Input: part model. Units: mm. Frame: model coordinates. A direction names the side the tool comes from. Round coordinates to 2 decimals unless told otherwise and drop trailing zeros. Order: outer loops, then holes, each group sorted by start corner. A loop starts at its lowest first (then second) coordinate and runs counter-clockwise, first axis right, second up. Notation, with made-up numbers: (86, -18.5) -> (139, -18.5) arc R28 cw to (139, 13.5) -> close; hole circle Ø2 at (44, 85.25). An arc over 180 degrees is marked (long way). Use a Markdown table: item, result.
from build123d import *

# Parameters (mm, degrees)
PAD_DEPTH            = 6.5
POCKET_DEPTH         = 6
SKETCH002_R          = 13.5
POCKET001_DEPTH      = 1
SKETCH003_W          = 5.45
SKETCH003_H          = 6.5
PAD001_DEPTH         = 3.5
POCKET002_DEPTH      = 10
SKETCH010_W          = 4
SKETCH010_H          = 6.5
PAD002_DEPTH         = 3.5
POCKET005_DEPTH      = 10
SKETCH015_R          = 2.2
SKETCH015_R_2        = 1.025
PAD003_DEPTH         = 2
POCKET009_DEPTH      = 4
POCKET010_DEPTH      = 4
PAD004_DEPTH         = 4
POCKET013_DEPTH      = 12.201
POCKET013_DEPTH_BACK = 36.201
SKETCH022_R          = 0.6
POCKET014_DEPTH      = 2
SKETCH023_R          = 0.6
POCKET015_DEPTH      = 2
SKETCH024_R          = 13.5
PAD005_DEPTH         = 1
SKETCH025_R          = 20.45
SKETCH025_R_2        = 19.85
POCKET016_DEPTH      = 0.3
SKETCH026_R          = 1
POCKET017_DEPTH      = 5
SKETCH027_W          = 5.4500000001
SKETCH027_H          = 2
SKETCH027_W_2        = 5.45
PAD006_DEPTH         = 2


with BuildPart() as part:
    # Sketch → Pad (new body)
    with BuildSketch(Plane.XY):
        with BuildLine():
            Line((-22.5019915649, 16), (-22.5019915649, -16))
            Line((-22.5019915649, -16), (-16.2858834578, -17.9))
            ThreePointArc((-16.2858834578, -17.9), (-0.4552796053, -24.1957169863), (15.6009615088, -18.5))
            Line((15.6009615088, -18.5), (24.5395016581, -17.45))
            Line((24.5395016581, 17.45), (24.5395016581, -17.45))
            Line((15.6009615088, 18.5), (24.5395016581, 17.45))
            ThreePointArc((15.6009615088, 18.5), (-0.4552796053, 24.1957169863), (-16.2858834578, 17.9))
            Line((-22.5019915649, 16), (-16.2858834578, 17.9))
        make_face()
    extrude(amount=PAD_DEPTH)

    # Sketch001 → Pocket (cut)
    with BuildSketch(Plane.XY):
        with BuildLine():
            Line((-14.8539557021, 16.9), (-21.2122180433, 15.55))
            Line((-21.2122180433, 15.55), (-21.2122180433, -15.55))
            Line((-21.2122180433, -15.55), (-14.8539557021, -16.9))
            ThreePointArc((-14.8539557021, -16.9), (-0.0760301383, -22.4998715423), (14.739402973, -17))
            Line((14.739402973, -17), (23.6191552218, -16.4))
            Line((23.6191552218, 16.4), (23.6191552218, -16.4))
            Line((14.739402973, 17), (23.6191552218, 16.4))
            ThreePointArc((14.739402973, 17), (-0.0760301383, 22.4998715423), (-14.8539557021, 16.9))
        make_face()
    extrude(amount=POCKET_DEPTH, mode=Mode.SUBTRACT)

    # Sketch002 (on Face19 of Pocket) → Pocket001 (cut)
    with BuildSketch(Plane(origin=(0, 0, 6), x_dir=(1, 0, 0), z_dir=(0, 0, -1))):
        Circle(SKETCH002_R)
    extrude(amount=-POCKET001_DEPTH, mode=Mode.SUBTRACT)

    # Sketch003 (on Face7 of Pad) → Pad001 (join)
    with BuildSketch(Plane.YZ.offset(24.5395016581)):
        with Locations((-14.725, 3.25)):
            Rectangle(SKETCH003_W, SKETCH003_H)
        with Locations((14.725, 3.25)):
            Rectangle(SKETCH003_W, SKETCH003_H)
    extrude(amount=PAD001_DEPTH)

    # Sketch006 (on Face22 of Pad001) → Pocket002 (cut)
    with BuildSketch(Plane.XY.offset(6.5)):
        with BuildLine():
            ThreePointArc((24.5395016581, 17.45), (26.1592830786, 16.2095505764), (28.0395016581, 15.4176006311))
            Line((28.0395016581, 17.45), (28.0395016581, 15.4176006311))
            Line((28.0395016581, 17.45), (24.5395016581, 17.45))
        make_face()
        with BuildLine():
            ThreePointArc((28.0395016581, -15.4176006311), (26.1592830786, -16.2095505765), (24.5395016581, -17.4500000001))
            Line((28.0395016581, -17.45), (24.5395016581, -17.4500000001))
            Line((28.0395016581, -15.4176006311), (28.0395016581, -17.45))
        make_face()
    extrude(amount=-POCKET002_DEPTH, mode=Mode.SUBTRACT)

    # Sketch010 (on Face3 of Pad) → Pad002 (join)
    with BuildSketch(Plane(origin=(-22.5019915649, 0, 0), x_dir=(0, -1, 0), z_dir=(-1, 0, 0))):
        with Locations((-14, 3.25)):
            Rectangle(SKETCH010_W, SKETCH010_H)
        with Locations((14, 3.25)):
            Rectangle(SKETCH010_W, SKETCH010_H)
    extrude(amount=PAD002_DEPTH)

    # Sketch011 (on Face28 of Pad002) → Pocket005 (cut)
    with BuildSketch(Plane.XY.offset(6.5)):
        Polygon((-26.0019915649, 16), (-22.5019915649, 16), (-26.0019915649, 14.5), align=None)
        Polygon((-22.5019915649, -16), (-26.0019915649, -14.5), (-26.0019915649, -16), align=None)
    extrude(amount=-POCKET005_DEPTH, mode=Mode.SUBTRACT)

    # Sketch015 (on Face19 of Pocket) → Pad003 (join)
    with BuildSketch(Plane(origin=(0, 0, 6), x_dir=(1, 0, 0), z_dir=(0, 0, -1))):
        with Locations((-18.42, 13.32)):
            Circle(SKETCH015_R)
        with Locations((-18.42, 13.32)):
            Circle(SKETCH015_R_2, mode=Mode.SUBTRACT)
        with Locations((7.27, 18.56)):
            Circle(SKETCH015_R)
        with Locations((7.27, 18.56)):
            Circle(SKETCH015_R_2, mode=Mode.SUBTRACT)
        with Locations((5.37, -19.79)):
            Circle(SKETCH015_R)
        with Locations((5.37, -19.79)):
            Circle(SKETCH015_R_2, mode=Mode.SUBTRACT)
        with Locations((-18.42, -13.32)):
            Circle(SKETCH015_R)
        with Locations((-18.42, -13.32)):
            Circle(SKETCH015_R_2, mode=Mode.SUBTRACT)
    extrude(amount=PAD003_DEPTH)

    # Sketch016 (on Face4 of Pocket) → Pocket009 (cut)
    with BuildSketch(Plane(origin=(0, 0, 0), x_dir=(1, 0, 0), z_dir=(0, 0, -1))):
        with BuildLine():
            Line((-4.9992330338, 23.6779996848), (-5.0007669662, 21.9372361465))
            ThreePointArc((5.0007669662, 21.9372361465), (0, 22.5), (-5.0007669662, 21.9372361465))
            Line((5.0007669662, 23.6776757675), (5.0007669662, 21.9372361465))
            ThreePointArc((5.0007669662, 23.6776757675), (0.00078388, 24.1999999873), (-4.9992330338, 23.6779996848))
        make_face()
    extrude(amount=-POCKET009_DEPTH, mode=Mode.SUBTRACT)

    # Sketch017 (on Face4 of Pocket) → Pocket010 (cut)
    with BuildSketch(Plane(origin=(0, 0, 0), x_dir=(1, 0, 0), z_dir=(0, 0, -1))):
        with BuildLine():
            ThreePointArc((-3.2541322314, -22.2634369184), (0, -22.5), (3.2541322314, -22.2634369184))
            Line((3.2541322314, -22.2634369184), (3.5, -23.9455632634))
            ThreePointArc((-3.5, -23.9455632634), (0, -24.2), (3.5, -23.9455632634))
            Line((-3.2541322314, -22.2634369184), (-3.5, -23.9455632634))
        make_face()
        with BuildLine():
            ThreePointArc((-13.9498796389, -17.6536358312), (-11.25, -19.4855715851), (-8.3135572795, -20.9077680626))
            Line((-8.3135572795, -20.9077680626), (-8.9416927184, -22.487466094))
            ThreePointArc((-15.0038705449, -18.987466094), (-12.1, -20.9578147716), (-8.9416927184, -22.487466094))
            Line((-13.9498796389, -17.6536358312), (-15.0038705449, -18.987466094))
        make_face()
        with BuildLine():
            ThreePointArc((8.3135572795, -20.9077680626), (11.25, -19.4855715851), (13.9498796389, -17.6536358312))
            Line((13.9498796389, -17.6536358312), (15.0038705449, -18.987466094))
            ThreePointArc((8.9416927184, -22.487466094), (12.1, -20.9578147716), (15.0038705449, -18.987466094))
            Line((8.3135572795, -20.9077680626), (8.9416927184, -22.487466094))
        make_face()
    extrude(amount=-POCKET010_DEPTH, mode=Mode.SUBTRACT)

    # Sketch018 (on Face8 of Pocket005) → Pad004 (join)
    with BuildSketch(Plane(origin=(0, 0, 0), x_dir=(1, 0, 0), z_dir=(0, 0, -1))):
        Polygon((-26.0019915649, 14.5), (-26.0019915649, 12), (-22.5019915649, 12), (-22.5019915649, 16), align=None)
        Polygon((-26.0019915649, -12), (-22.5019915649, -12), (-22.5019915649, -16), (-26.0019915649, -14.5), align=None)
        with BuildLine():
            Line((24.5395016581, 17.4500000001), (24.5395016581, 12))
            Line((28.0395016581, 12), (24.5395016581, 12))
            Line((28.0395016581, 15.4176006311), (28.0395016581, 12))
            ThreePointArc((24.5395016581, 17.4500000001), (26.1592830786, 16.2095505765), (28.0395016581, 15.4176006311))
        make_face()
        with BuildLine():
            Line((24.5395016581, -12), (24.5395016581, -17.45))
            ThreePointArc((28.0395016581, -15.4176006311), (26.1592830786, -16.2095505764), (24.5395016581, -17.45))
            Line((28.0395016581, -12), (28.0395016581, -15.4176006311))
            Line((24.5395016581, -12), (28.0395016581, -12))
        make_face()
    extrude(amount=PAD004_DEPTH)

    # Sketch021 (on Face50 of Pad004) → Pocket013 (cut, two sides)
    with BuildSketch(Plane(origin=(0, -12, 0), x_dir=(-1, 0, 0), z_dir=(0, 1, 0))) as pocket013_sk:
        with BuildLine():
            Line((-24.5395016581, -4), (-24.5395016581, -3))
            ThreePointArc((-25.5395016581, -4), (-24.958362828, -3.5811388301), (-24.5395016581, -3))
            Line((-24.5395016581, -4), (-25.5395016581, -4))
        make_face()
        with BuildLine():
            Line((22.5019915649, -4), (22.5019915649, -3))
            ThreePointArc((22.5019915649, -3), (22.9208527349, -3.5811388301), (23.5019915649, -4))
            Line((22.5019915649, -4), (23.5019915649, -4))
        make_face()
        with BuildLine():
            Line((-28.0395016581, 0), (-28.0395016581, 6.5))
            Line((-28.0395016581, 6.5), (-24.5395016581, 6.5))
            ThreePointArc((-24.5395016581, 6.5), (-27.1088837932, 3.6912057651), (-28.0395016581, 0))
        make_face()
        with BuildLine():
            Line((26.0019915649, 6.5), (26.0019915649, 0))
            ThreePointArc((26.0019915649, 0), (25.0713737, 3.6912057651), (22.5019915649, 6.5))
            Line((26.0019915649, 6.5), (22.5019915649, 6.5))
        make_face()
    extrude(amount=-POCKET013_DEPTH, mode=Mode.SUBTRACT)
    extrude(pocket013_sk.sketch, amount=POCKET013_DEPTH_BACK, mode=Mode.SUBTRACT)

    # Sketch022 (on Face66 of Pocket013) → Pocket014 (cut)
    with BuildSketch(Plane.XZ.offset(-12)):
        with Locations((-24.7019915649, -2.7)):
            Circle(SKETCH022_R)
        with Locations((26.7395016581, -2.7)):
            Circle(SKETCH022_R)
    extrude(amount=-POCKET014_DEPTH, mode=Mode.SUBTRACT)

    # Sketch023 (on Face49 of Pocket014) → Pocket015 (cut)
    with BuildSketch(Plane(origin=(0, -12, 0), x_dir=(-1, 0, 0), z_dir=(0, 1, 0))):
        with Locations((-26.7395016581, -2.7)):
            Circle(SKETCH023_R)
        with Locations((24.7019915649, -2.7)):
            Circle(SKETCH023_R)
    extrude(amount=-POCKET015_DEPTH, mode=Mode.SUBTRACT)

    # Sketch024 (on Face16 of Pocket015) → Pad005 (join)
    with BuildSketch(Plane.XY.offset(6.5)):
        with BuildLine():
            ThreePointArc((-22.5019915649, -8.9050758341), (24.2, 0), (-22.5019915649, 8.9050758341))
            Line((-22.5019915649, 8.9050758341), (-22.5019915649, -8.9050758341))
        make_face()
        Circle(SKETCH024_R, mode=Mode.SUBTRACT)
    extrude(amount=PAD005_DEPTH)

    # Sketch025 (on Face42 of Pad005) → Pocket016 (cut)
    with BuildSketch(Plane.XY.offset(7.5)):
        Circle(SKETCH025_R)
        Circle(SKETCH025_R_2, mode=Mode.SUBTRACT)
    extrude(amount=-POCKET016_DEPTH, mode=Mode.SUBTRACT)

    # Sketch026 (on DatumPlane) → Pocket017 (cut)
    with BuildSketch(Plane.XZ.offset(25)):
        with Locations((-6.5, 4.8)):
            Circle(SKETCH026_R)
    extrude(amount=-POCKET017_DEPTH, mode=Mode.SUBTRACT)

    # Sketch027 (on Face18 of Pocket017) → Pad006 (join)
    with BuildSketch(Plane(origin=(24.5395016581, 0, 0), x_dir=(0, -1, 0), z_dir=(-1, 0, 0))):
        with Locations((14.7250000001, -2)):
            Rectangle(SKETCH027_W, SKETCH027_H)
        with Locations((-14.725, -2)):
            Rectangle(SKETCH027_W_2, SKETCH027_H)
    extrude(amount=PAD006_DEPTH)


solid = part.part
1) Set-up query: faces 1 (the face through (-8.623, 21.687, 1.972)), 2 (the face through (4.61, 19.1, 5.01)), 3 (the face through (-17, 11, 7.2)), 4 (the face through (22.54, 15, -2)), 5 (the face through (-14.47, 18.31, 1.97)). Return all of +Z, -Z, +X, -X, +Y, -Y with unobstructed straight access to the full face (end or side cutting, diameter ignored); none if empty.
Answer key:
| item | result |
|---|---|
| face 1 | -Z, -X |
| face 2 | -Z |
| face 3 | +Z |
| face 4 | -Z, +Y, -Y |
| face 5 | -Z, +Y |
2) Cut plane B-B on y = -3. Return loops of the section in (x, z), and give its area (3 significant figures).
Answer key:
| item | result |
|---|---|
| outline | (-22.5, 0) -> (-21.21, 0) -> (-21.21, 6) -> (-13.16, 6) -> (-13.16, 7.5) -> (-19.62, 7.5) -> (-19.62, 7.2) -> (-20.23, 7.2) -> (-20.23, 7.5) -> (-22.5, 7.5) -> close; (13.16, 6) -> (23.62, 6) -> (23.62, 0) -> (24.54, 0) -> (24.54, 6.5) -> (24.01, 6.5) -> (24.01, 7.5) -> (20.23, 7.5) -> (20.23, 7.2) -> (19.62, 7.2) -> (19.62, 7.5) -> (13.16, 7.5) -> close |
| area | 43.4 mm^2 |
3) Ray query, probe 1 along Y at (x, z) = (7.27, 5) (3 decimals); probe 2 along Y at (x, z) = (0, 7.4); probe 3 along X at (y, z) = (0.5, 5.5). Return the intervals inside material, ascending.
Answer key:
| item | result |
|---|---|
| probe 1 | y = -23.082 to -21.293, -20.76 to -19.585, -17.535 to -16.36, 18.681 to 20.899, 21.293 to 23.082 |
| probe 2 | y = -24.2 to -20.45, -19.85 to -13.5, 13.5 to 19.85, 20.45 to 24.2 |
| probe 3 | x = -22.5 to -21.21, 23.62 to 24.54 |
4) Cut plane C-C on z = 1.5. State how many separate pieces and enclosed holes the cut face has, and give its area (3 significant figures).
Answer key:
| item | result |
|---|---|
| separate pieces | 4 |
| enclosed holes | 0 |
| area | 223 mm^2 |
5) Cut plane A-A on x = 0. Return loops of the section in (y, z).
Answer key:
| item | result |
|---|---|
| outline | (-24.2, 4) -> (-22.5, 4) -> (-22.5, 6) -> (-13.5, 6) -> (-13.5, 7.5) -> (-19.85, 7.5) -> (-19.85, 7.2) -> (-20.45, 7.2) -> (-20.45, 7.5) -> (-24.2, 7.5) -> close; (13.5, 6) -> (22.5, 6) -> (22.5, 4) -> (24.2, 4) -> (24.2, 7.5) -> (20.45, 7.5) -> (20.45, 7.2) -> (19.85, 7.2) -> (19.85, 7.5) -> (13.5, 7.5) -> close |
6) Cut plane D-D on x = 17. Return loops of the section in (y, z).
Answer key:
| item | result |
|---|---|
| outline | (-18.34, 0) -> (-16.85, 0) -> (-16.85, 6) -> (16.85, 6) -> (16.85, 0) -> (18.34, 0) -> (18.34, 6.5) -> (17.22, 6.5) -> (17.22, 7.5) -> (11.37, 7.5) -> (11.37, 7.2) -> (10.25, 7.2) -> (10.25, 7.5) -> (-10.25, 7.5) -> (-10.25, 7.2) -> (-11.37, 7.2) -> (-11.37, 7.5) -> (-17.22, 7.5) -> (-17.22, 6.5) -> (-18.34, 6.5) -> close |
7) Contact query for flat-ended pins moving along their axis: P1, Ø2.5, axis at x = -6.5, z = 4.8, coming from the -Y side; P2, Ø2.5, axis at x = 6.5, y = 21.5, coming from the -Z side; P3, Ø4, axis at x = 11, y = 19, coming from the -Z side. Output: stop coordinate, or through.
Answer key:
| item | result |
|---|---|
| P1 | stops at y = -23.62 |
| P2 | stops at z = 0 |
| P3 | stops at z = 4 |
